Source: CAD feature listing. Evaluate the final solid. Frame: model axes, mm. Face numbers are marked on the shaded views. A direction names the side the tool comes from. Round coordinates to 2 decimals unless told otherwise and drop trailing zeros. Order: outer loops, then holes, each group sorted by start corner. A loop starts at its lowest first (then second) coordinate and runs counter-clockwise, first axis right, second up. Notation, with made-up numbers: M 59.25,-21 L 113.25,-21 A31 cw 113.25,11 Z; hole C -24.5,-4 d8. An arc over 180 degrees is marked long. Use one line per item in the form item = value. Start each with the question number.
Q1. Section B-B (x = 0). Return the cut outline in (y, z), plus the area to 3 significant figures.
Q2. Pull-direction query (Z, two-part tool) for the marked faces 1, 2 and 3; classes: pulls with the +Z half, pulls with the -Z half, needs draft (parallel to the pull), parting line crosses it, or undercut.
Q3. Section A-A (z = 0). Return the cut outline in (x, y).
Q4. Section C-C (y = -15). Return the cut outline in (x, z).
Q5. Material intervals for probe 1 along Z at (x, y) = (-4.5, 2.5); probe 2 along Z at (x, y) = (0, -4.5); probe 3 along Y at (x, z) = (-8, 49), sorted ascending.
Q6. Contact query for flat-ended pins moving along their axis: pin 1 (4 mm diameter, centred on x = 26, y = -27, fed in from -Z); pin 2 (1.5 mm diameter, centred on y = -5.5, z = 5, fed in from +X); pin 3 (10 mm diameter, centred on x = -9.5, y = -11.5, fed in from -Z). Output: stop coordinate, or through.
Q7. Reachability of the marked faces 4 and 5 from +Z, -Z, +X, -X, +Y, -Y: full face, straight path, thin tool, end or side. Return the list, or none.
from build123d import *

# Parameters (mm, degrees)
F0_R            = 69.85
F1_DEPTH        = 19.05
F2_R            = 35.052
F3_DEPTH        = 34.798
F4_R            = 19.0246
F5_DEPTH        = 53.849
F6_R            = 6.35
F7_DEPTH        = 19.051
F7_COPIES_COUNT = 4
F8_R            = 3.048


# Not quite as in the source:
# - a pattern or mirror of a feature is missing from the dataset's text; its kind, count and spacing are read off the source's solid


with BuildPart() as f1:
    # F0 (on Front) → F1 (new body)
    with BuildSketch(Plane.XZ):
        Circle(F0_R)
    extrude(amount=-F1_DEPTH)

    # F2 (on face) → F3 (join)
    with BuildSketch(Plane.XZ):
        Circle(F2_R)
    extrude(amount=F3_DEPTH)

    # F4 (on face) → F5 (cut, through all)
    with BuildSketch(Plane.XZ.offset(34.798)):
        Circle(F4_R)
    extrude(amount=-F5_DEPTH, mode=Mode.SUBTRACT)

    # F6 (on face) → F7 (cut, through all)
    with BuildSketch(Plane.XZ):
        with Locations((0, 53.848)):
            Circle(F6_R)
    f7 = extrude(amount=-F7_DEPTH, mode=Mode.SUBTRACT)

    # F7_copies: F7 ×4 about axis
    f7_copies_axis = Axis((0, 0, 0), (0, 1, 0))
    for i in range(1, F7_COPIES_COUNT):
        add(f7.rotate(f7_copies_axis, i * 360 / F7_COPIES_COUNT), mode=Mode.SUBTRACT)

    # F8
    f8_edges = [f1.edges().sort_by_distance(p)[0] for p in [
        (-35.052, -34.798, 0),
        (-35.052, 0, 0),
        (-69.85, 0, 0),
    ]]
    fillet(f8_edges, radius=F8_R)


solid = f1.part
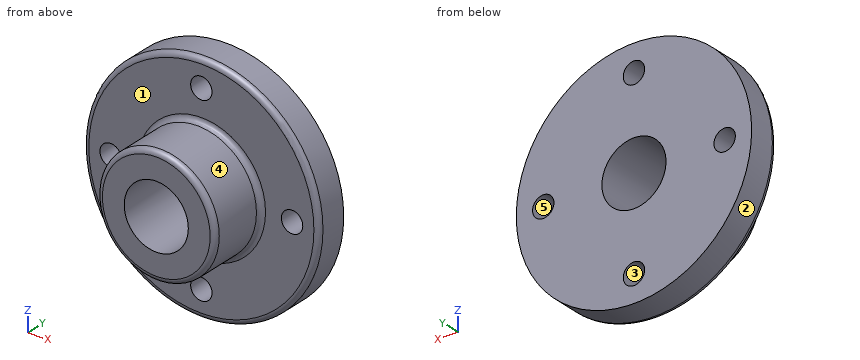
Results list:
q1.outline = M -34.8,-32 A3.05 ccw -31.75,-35.05 L -3.05,-35.05 A3.05 cw 0,-38.1 L 0,-47.5 L 19.05,-47.5 L 19.05,-19.02 L -34.8,-19.02 Z; M -34.8,19.02 L 19.05,19.02 L 19.05,47.5 L 0,47.5 L 0,38.1 A3.05 cw -3.05,35.05 L -31.75,35.05 A3.05 ccw -34.8,32 Z; M 0,-66.8 A3.05 ccw 3.05,-69.85 L 19.05,-69.85 L 19.05,-60.2 L 0,-60.2 Z; M 0,60.2 L 19.05,60.2 L 19.05,69.85 L 3.05,69.85 A3.05 ccw 0,66.8 Z
q1.area = 2,560 mm2
q2.face_1 = needs draft
q2.face_2 = parting line crosses it
q2.face_3 = undercut
q3.outline = M -69.85,3.05 A3.05 ccw -66.8,0 L -60.2,0 L -60.2,19.05 L -69.85,19.05 Z; M -47.5,0 L -38.1,0 A3.05 cw -35.05,-3.05 L -35.05,-31.75 A3.05 ccw -32,-34.8 L -19.02,-34.8 L -19.02,19.05 L -47.5,19.05 Z; M 19.02,-34.8 L 32,-34.8 A3.05 ccw 35.05,-31.75 L 35.05,-3.05 A3.05 cw 38.1,0 L 47.5,0 L 47.5,19.05 L 19.02,19.05 Z; M 60.2,0 L 66.8,0 A3.05 ccw 69.85,3.05 L 69.85,19.05 L 60.2,19.05 Z
q4.outline = C 0,0 d70.1; hole C 0,0 d38.05
q5.probe_1 = -69.66 to -58.33, -49.37 to -18.48, 18.48 to 49.37, 58.33 to 69.66
q5.probe_2 = -35.05 to -19.02, 19.02 to 35.05
q5.probe_3 = 0 to 19.05
q6.pin_1 = -25.55
q6.pin_2 = 34.79
q6.pin_3 = -34.76
q7.face_4 = -Y
q7.face_5 = +Y, -Y
